```python
from build123d import *

# Parameters (mm, degrees)
SKETCH_1_W      = 20
SKETCH_1_H      = 3
EXTRUDE_1_DEPTH = 3


with BuildPart() as part:
    # Эскиз1 → Бобышка-Вытянуть1 (new body)
    with BuildSketch(Plane(origin=(0, 0, 0), x_dir=(0, 0, -1), z_dir=(1, 0, 0))):
        Polygon((-118, -165), (-118, -145.2), (-121, -145.2), (-121, -124.8), (-118, -124.8), (-118, -75.2), (-121, -75.2), (-121, -54.8), (-118, -54.8), (-118, -5.2), (-121, -5.2), (-121, 15.2), (-118, 15.2), (-118, 64.8), (-121, 64.8), (-121, 85.2), (-118, 85.2), (-118, 134.8), (-121, 134.8), (-121, 155.2), (-118, 155.2), (-118, 165), (118, 165), (118, 155.2), (121, 155.2), (121, 134.8), (118, 134.8), (118, 85.2), (121, 85.2), (121, 64.8), (118, 64.8), (118, 15.2), (121, 15.2), (121, -5.2), (118, -5.2), (118, -54.8), (121, -54.8), (121, -75.2), (118, -75.2), (118, -124.8), (121, -124.8), (121, -145.2), (118, -145.2), (118, -165), align=None)
        with Locations((-64, -85.5)):
            Rectangle(SKETCH_1_W, SKETCH_1_H, mode=Mode.SUBTRACT)
        with Locations((0, -85.5)):
            Rectangle(SKETCH_1_W, SKETCH_1_H, mode=Mode.SUBTRACT)
        with Locations((64, -85.5)):
            Rectangle(SKETCH_1_W, SKETCH_1_H, mode=Mode.SUBTRACT)
    extrude(amount=EXTRUDE_1_DEPTH)


solid = part.part
```
Geometry: final body of the model. Coordinates: model frame, mm. Coordinates: 2 decimals unless noted, no trailing zeros. Order: outer loops, then holes, each group sorted by start corner. A loop starts at its lowest first (then second) coordinate and runs counter-clockwise, first axis right, second up. Notation, with made-up numbers: (-3, -39.75) - (11, -39.75) arc R25 ccw to (11, -25.75) - close; hole circle Ø3 at (26.5, 39.5). An arc over 180 degrees is marked (long way). Return JSON: item names as keys, results as strings. Group by question number.
1. Cut plane A-A (y = -118.5). Output: boundary loops of the cut face in (x, z).
2. Cut plane B-B (x = 2.3). Count the separate pieces of the cut face and the enclosed holes in it, plus the area to 3 significant figures.
3. Material intervals for line 1 along Y through (x, z) = (0.5, 66); line 2 along Z through (x, y) = (2.4, 36.5), sorted ascending. Write a range as [from, to].
4. Pin query (flat end, axial travel): pin 1 (0.9 mm diameter, centred on x = 1, y = -85.5, fed in from -Z); pin 2 (0.9 mm diameter, centred on x = 1, z = -120, fed in from +Y); pin 3 (1.5 mm diameter, centred on x = 2, z = 119, fed in from -Y); pin 4 (4 mm diameter, centred on y = -73.5, z = -71.5, fed in from -X). Return the tip coordinate at first contact, or that it passes through.
Resolved:
{
 "1": {"outline": "(0, -118) - (3, -118) - (3, 118) - (0, 118) - close"},
 "2": {"separate pieces": "1", "enclosed holes": "3", "area": "78,300 mm²"},
 "3": {"line 1": "y = [-165, -87], [-84, 165]", "line 2": "z = [-118, 118]"},
 "4": {"pin 1": "stops at z = -118", "pin 2": "stops at y = 155.2", "pin 3": "stops at y = -145.2", "pin 4": "stops at x = 0"}
}
